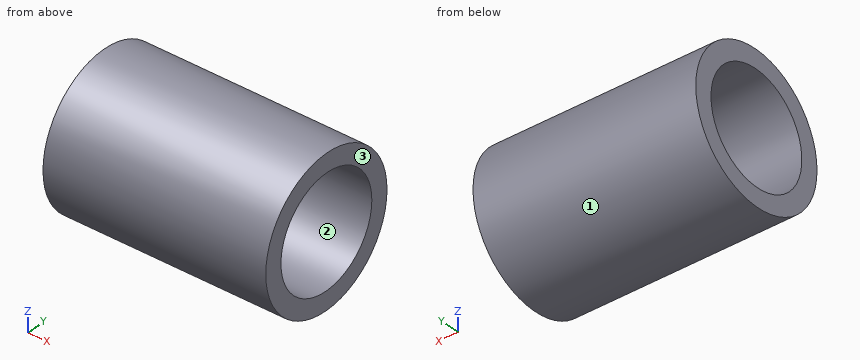
from build123d import *

# Parameters (mm, degrees)
SKETCH1_W = 12
SKETCH1_H = 4


with BuildPart() as part:
    # Sketch1 → Revolve1 (revolve)
    with BuildSketch(Plane.XY, mode=Mode.PRIVATE) as revolve1_sk:
        with Locations((6, 2)):
            Rectangle(SKETCH1_W, SKETCH1_H)
    revolve(revolve1_sk.sketch.rotate(Axis((0, 0, 0), (1, 0, 0)), 90), axis=Axis((0, 0, 0), (1, 0, 0)))

    # SurfaceCut1: cut with a surface, the side it looks to stays
    # Surface-Revolve1: a surface, the sketch's curves turned about an axis
    with BuildLine(Plane.XY, mode=Mode.PRIVATE) as surface_revolve1_1_path:
        Line((0, 3), (12, 3))
    surface_revolve1_1 = Shell.revolve(surface_revolve1_1_path.wire(), 360, Axis((0, 0, 0), (1, 0, 0)))
    split(bisect_by=surface_revolve1_1, keep=Keep.TOP)


solid = part.part
Geometry: final body of the model. Coordinates: model frame, mm. Face numbers are marked on the shaded views. Give positions to 0.01 mm unless a question says otherwise; leave off trailing zeros. Order: outer loops, then holes, each group sorted by start corner. A loop starts at its lowest first (then second) coordinate and runs counter-clockwise, first axis right, second up. Notation, with made-up numbers: (19, 39.25) -> (71, 39.25) arc R6 cw to (71, 48.25) -> close; hole circle Ø7 at (18, 85). An arc over 180 degrees is marked (long way). Put each result on its own line as item: value.
Q1. Draft query along Z for the marked faces 1, 2 and 3. Return one class per face: released by +Z, released by -Z, zero draft, split by the parting line, or undercut.
Here are the results:
face 1: split by the parting line
face 2: undercut
face 3: zero draft
Q2. Material intervals for L1, parallel to Y at x = 3.5, z = -0.25; L2, parallel to Y at x = 5.75, z = 1.25; L3, parallel to Z at x = 11, y = -2, sorted ascending.
Here are the results:
L1: y = -3.99 to -2.99, 2.99 to 3.99
L2: y = -3.8 to -2.73, 2.73 to 3.8
L3: z = -3.46 to -2.24, 2.24 to 3.46
Q3. Section C-C, the plane x = 9.25. Return loops of the section in (y, z).
Here are the results:
outline: circle Ø8 at (0, 0); hole circle Ø6 at (0, 0)
Q4. Pin query (flat end, axial travel): pin 1 (3 mm diameter, centred on x = 2, z = 1.5, fed in from -Y); pin 2 (2 mm diameter, centred on y = -1.5, z = 0, fed in from -X) (3 decimals); pin 3 (1.5 mm diameter, centred on x = 9.5, y = -3, fed in from +Z). Return the tip coordinate at first contact, or that it passes through.
Here are the results:
pin 1: stops at y = -4
pin 2: passes through
pin 3: stops at z = 3.31
Q5. Section A-A, the plane y = 0. Return loops of the section in (x, z), then the cut area to 3 significant figures.
Here are the results:
outline: (0, -4) -> (12, -4) -> (12, -3) -> (0, -3) -> close; (0, 3) -> (12, 3) -> (12, 4) -> (0, 4) -> close
area: 24.0 mm^2
